Autodesk Inventor part; units mm, degrees
ref_plane "YZ Plane" through (0, 0, 0) normal (1, 0, 0) x (0, 1, 0)
ref_plane "XZ Plane" through (0, 0, 0) normal (0, 1, 0) x (-1, 0, 0)
ref_plane "XY Plane" through (0, 0, 0) normal (0, 0, 1) x (1, 0, 0)
sketch "Sketch1" plane through (0, 0, 0) normal (0, 0, 1) x (1, 0, 0)
  line L0 (0, 0) -> (127, 0)
  line L1 (127, 0) -> (127, 127)
  line L2 (127, 127) -> (0, 127)
  line L3 (0, 127) -> (0, 0)
  circle A0 centre (63.5, 63.5) radius 12.6844 construction
  circle A1 centre (9.4388, 90.7552) radius 3.175
  circle A2 centre (117.5612, 90.7552) radius 3.175
  circle A3 centre (117.5612, 36.2448) radius 3.175
  circle A4 centre (9.4388, 36.2448) radius 3.175
  line L4 (9.4388, 90.7552) -> (117.5612, 36.2448) construction
  line L5 (50.8, 50.8) -> (76.2, 50.8)
  line L6 (76.2, 50.8) -> (76.2, 76.2)
  line L7 (76.2, 76.2) -> (50.8, 76.2)
  line L8 (50.8, 76.2) -> (50.8, 50.8)
  line L9 (50.8, 50.8) -> (76.2, 76.2) construction
  line L10 (76.2, 50.8) -> (50.8, 76.2) construction
  point P0 (63.5, 127)
  point P1 (127, 63.5)
  dimension "d0" = 127
  dimension "d1" = 127
  dimension "d2" = 6.35
  dimension "d6" = 25.4
  dimension "d7" = 25.4
extrude "Extrusion1" add sketch "Sketch1" along normal blind 25.4
sketch "Sketch2" plane through (0, 0, 25.4) normal (0, 0, 1) x (1, 0, 0)
  line L0 (50.8, 50.8) -> (50.8, 76.2)
  line L1 (19.05, 76.2) -> (50.8, 76.2)
  line L2 (50.8, 76.2) -> (50.8, 69.85)
  line L3 (50.8, 69.85) -> (19.05, 69.85)
  line L4 (19.05, 69.85) -> (19.05, 76.2)
  line L5 (19.05, 57.15) -> (50.8, 57.15)
  line L6 (50.8, 57.15) -> (50.8, 50.8)
  line L7 (50.8, 50.8) -> (19.05, 50.8)
  line L8 (19.05, 50.8) -> (19.05, 57.15)
  line L9 (19.05, 67.31) -> (38.1, 67.31)
  line L10 (38.1, 67.31) -> (38.1, 59.69)
  line L11 (38.1, 59.69) -> (19.05, 59.69)
  line L12 (19.05, 59.69) -> (19.05, 67.31)
  line L13 (50.8, 76.2) -> (76.2, 76.2)
  line L14 (0, 127) -> (0, 0)
  line L15 (127, 127) -> (0, 127)
  line L16 (63.5, 127) -> (63.5, 0) construction
  line L17 (0, 0) -> (127, 0)
  line L18 (76.2, 50.8) -> (76.2, 76.2)
  line L19 (107.95, 76.2) -> (76.2, 76.2)
  line L20 (76.2, 76.2) -> (76.2, 69.85)
  line L21 (76.2, 69.85) -> (107.95, 69.85)
  line L22 (107.95, 69.85) -> (107.95, 76.2)
  line L23 (107.95, 57.15) -> (76.2, 57.15)
  line L24 (76.2, 57.15) -> (76.2, 50.8)
  line L25 (76.2, 50.8) -> (107.95, 50.8)
  line L26 (107.95, 50.8) -> (107.95, 57.15)
  line L27 (107.95, 67.31) -> (88.9, 67.31)
  line L28 (88.9, 67.31) -> (88.9, 59.69)
  line L29 (88.9, 59.69) -> (107.95, 59.69)
  line L30 (107.95, 59.69) -> (107.95, 67.31)
  line L31 (127, 127) -> (127, 0)
  point P0 (50.8, 76.2)
  dimension "d8" = 6.35
  dimension "d9" = 6.35
  dimension "d10" = 2.54
  dimension "d11" = 2.54
  dimension "d12" = 12.7
  dimension "d13" = 19.05
extrude "Extrusion2" cut sketch "Sketch2" against normal blind 25.4 contours L7 L8 L5 L0 | L23 L26 L25 L18 | L19 L22 L21 L18 | L3 L4 L1 L0 | L9 L10 L11 L12 | L30 L29 L28 L27
sketch "Sketch4" plane through (0, 0, 25.4) normal (0, 0, 1) x (1, 0, 0)
  line L0 (6.35, 82.55) -> (15.875, 82.55)
  line L1 (15.875, 82.55) -> (15.875, 44.45)
  line L2 (15.875, 44.45) -> (6.35, 44.45)
  line L3 (6.35, 44.45) -> (6.35, 82.55)
  line L4 (0, 127) -> (0, 0)
  line L5 (19.05, 69.85) -> (19.05, 76.2)
  line L6 (127, 127) -> (0, 127)
  line L7 (63.5, 127) -> (63.5, 0) construction
  line L8 (0, 0) -> (127, 0)
  line L9 (120.65, 82.55) -> (111.125, 82.55)
  line L10 (111.125, 82.55) -> (111.125, 44.45)
  line L11 (111.125, 44.45) -> (120.65, 44.45)
  line L12 (120.65, 44.45) -> (120.65, 82.55)
  line L13 (127, 127) -> (127, 0)
  line L14 (107.95, 69.85) -> (107.95, 76.2)
  point P0 (6.35, 63.5)
  point P1 (0, 63.5)
  point P2 (120.65, 63.5)
  dimension "d25" = 38.1
  dimension "d27" = 3.175
  dimension "d28" = 6.35
extrude "Extrusion4" cut sketch "Sketch4" against normal blind 25.4 contours L0 L1 L2 L3 | L12 L11 L10 L9
sketch "Sketch3" plane through (0, 0, 25.4) normal (0, 0, 1) x (1, 0, 0)
  line L0 (19.05, 50.8) -> (107.95, 50.8)
  line L1 (44.45, 50.8) -> (50.8, 50.8)
  line L2 (50.8, 50.8) -> (50.8, 19.05)
  line L3 (50.8, 19.05) -> (44.45, 19.05)
  line L4 (44.45, 19.05) -> (44.45, 50.8)
  line L5 (76.2, 50.8) -> (82.55, 50.8)
  line L6 (82.55, 50.8) -> (82.55, 19.05)
  line L7 (82.55, 19.05) -> (76.2, 19.05)
  line L8 (76.2, 19.05) -> (76.2, 50.8)
  line L9 (53.975, 38.1) -> (73.025, 38.1)
  line L10 (73.025, 38.1) -> (73.025, 19.05)
  line L11 (73.025, 19.05) -> (53.975, 19.05)
  line L12 (53.975, 19.05) -> (53.975, 38.1)
  line L13 (0, 0) -> (127, 0)
  line L14 (0, 127) -> (0, 0)
  line L15 (0, 63.5) -> (127, 63.5) construction
  line L16 (44.45, 76.2) -> (50.8, 76.2)
  line L17 (50.8, 76.2) -> (50.8, 107.95)
  line L18 (50.8, 107.95) -> (44.45, 107.95)
  line L19 (44.45, 107.95) -> (44.45, 76.2)
  line L20 (76.2, 76.2) -> (82.55, 76.2)
  line L21 (82.55, 76.2) -> (82.55, 107.95)
  line L22 (82.55, 107.95) -> (76.2, 107.95)
  line L23 (76.2, 107.95) -> (76.2, 76.2)
  line L24 (53.975, 88.9) -> (73.025, 88.9)
  line L25 (73.025, 88.9) -> (73.025, 107.95)
  line L26 (73.025, 107.95) -> (53.975, 107.95)
  line L27 (53.975, 107.95) -> (53.975, 88.9)
  point P0 (63.5, 19.05)
  point P1 (63.5, 50.8)
  point P2 (63.5, 107.95)
  point P3 (63.5, 76.2)
  dimension "d16" = 19.05
  dimension "d17" = 3.175
  dimension "d18" = 3.175
  dimension "d19" = 19.05
  dimension "d20" = 6.35
  dimension "d21" = 6.35
  dimension "d22" = 12.7
extrude "Extrusion3" cut sketch "Sketch3" against normal blind 25.4
sketch "Sketch5" plane through (0, 0, 25.4) normal (0, 0, 1) x (1, 0, 0)
  line L0 (41.275, 15.875) -> (85.725, 15.875)
  line L1 (85.725, 15.875) -> (85.725, 6.35)
  line L2 (85.725, 6.35) -> (41.275, 6.35)
  line L3 (41.275, 6.35) -> (41.275, 15.875)
  line L4 (0, 127) -> (0, 0)
  line L5 (0, 63.5) -> (127, 63.5) construction
  line L6 (127, 0) -> (127, 127)
  line L7 (73.025, 19.05) -> (53.975, 19.05)
  line L8 (0, 0) -> (127, 0)
  line L9 (41.275, 111.125) -> (85.725, 111.125)
  line L10 (85.725, 111.125) -> (85.725, 120.65)
  line L11 (85.725, 120.65) -> (41.275, 120.65)
  line L12 (41.275, 120.65) -> (41.275, 111.125)
  point P0 (63.5, 6.35)
  point P1 (63.5, 0)
  point P2 (63.5, 120.65)
  point P3 (63.5, 127)
  dimension "d31" = 3.175
  dimension "d32" = 6.35
  dimension "d33" = 44.45
extrude "Extrusion5" cut sketch "Sketch5" against normal blind 25.4
properties part number "BearingFlexure"
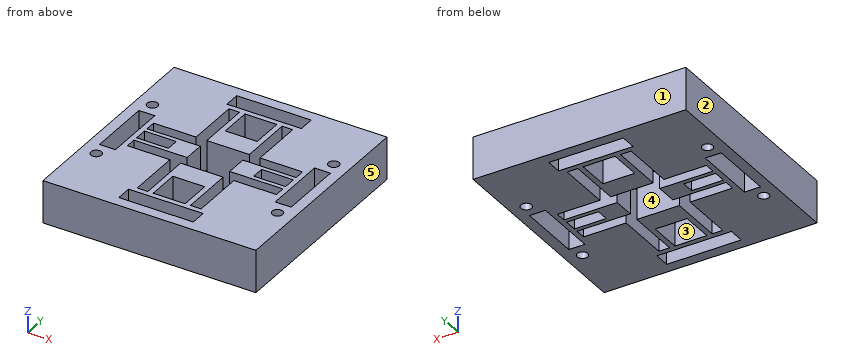
CAD build for the part. Positions are in the model's coordinates, mm. Face numbers are marked on the shaded views. A direction names the side the tool comes from. Round coordinates to 2 decimals unless told otherwise and drop trailing zeros. Write each loop counter-clockwise with the first axis right and the second up, starting at its lowest first coordinate (ties: lowest second). Pieces come first, ordered by that corner, then holes. Notation, with made-up numbers: (48.5, 36.5) -> (102.5, 36.5) arc R31 ccw to (102.5, 72.5) -> close; hole circle Ø4 at (34.5, 24). An arc over 180 degrees is marked (long way). Answer as a JSON object with one key per item and string values.
(1) Two-plate mould, pull along X, no slides. Class the marked faces 1, 2 and 3: +X half, -X half, draft (parallel to the pull), parting line (faces both ways), or undercut.
Reported:
{"face 1": "draft", "face 2": "-X half", "face 3": "undercut"}
(2) Probe probe 1 along X at (y, z) = (43, 21); probe 2 along Y at (x, z) = (62.5, 10) (3 decimals); probe 3 along Y at (x, z) = (29, 20). List the from-to ranges inside material, lowest first. Write a range as [from, to].
Reported:
{"probe 1": "x = [0, 44.45], [50.8, 76.2], [82.55, 127]", "probe 2": "y = [0, 6.35], [15.875, 19.05], [38.1, 50.8], [76.2, 88.9], [107.95, 111.125], [120.65, 127]", "probe 3": "y = [0, 50.8], [57.15, 59.69], [67.31, 69.85], [76.2, 127]"}
(3) Band-saw the part on D-D, the plane x = 21. List the corners of the cut face in (y, z).
Reported:
{"outline": "(0, 0) -> (50.8, 0) -> (50.8, 25.4) -> (0, 25.4) -> close; (57.15, 0) -> (59.69, 0) -> (59.69, 25.4) -> (57.15, 25.4) -> close; (67.31, 0) -> (69.85, 0) -> (69.85, 25.4) -> (67.31, 25.4) -> close; (76.2, 0) -> (127, 0) -> (127, 25.4) -> (76.2, 25.4) -> close"}
(4) Band-saw the part on A-A, the plane y = 63.5. List the corners of the cut face in (x, z) (3 decimals), then the cut area to 3 significant figures.
Reported:
{"outline": "(0, 0) -> (6.35, 0) -> (6.35, 25.4) -> (0, 25.4) -> close; (15.875, 0) -> (19.05, 0) -> (19.05, 25.4) -> (15.875, 25.4) -> close; (38.1, 0) -> (50.8, 0) -> (50.8, 25.4) -> (38.1, 25.4) -> close; (76.2, 0) -> (88.9, 0) -> (88.9, 25.4) -> (76.2, 25.4) -> close; (107.95, 0) -> (111.125, 0) -> (111.125, 25.4) -> (107.95, 25.4) -> close; (120.65, 0) -> (127, 0) -> (127, 25.4) -> (120.65, 25.4) -> close", "area": "1,130 mm^2"}
(5) Band-saw the part on C-C, the plane y = 99.5. List the corners of the cut face in (x, z) (3 decimals).
Reported:
{"outline": "(0, 0) -> (44.45, 0) -> (44.45, 25.4) -> (0, 25.4) -> close; (50.8, 0) -> (53.975, 0) -> (53.975, 25.4) -> (50.8, 25.4) -> close; (73.025, 0) -> (76.2, 0) -> (76.2, 25.4) -> (73.025, 25.4) -> close; (82.55, 0) -> (127, 0) -> (127, 25.4) -> (82.55, 25.4) -> close"}
(6) Which spindle directions (+Z, -Z, +X, -X, +Y, -Y) get a long thin tool onto all of the face, cutting with end or side? Do the marked faces 4 and 5. Say none if no direction does.
Reported:
{"face 4": "+Z, -Z", "face 5": "+Z, -Z, +X, +Y, -Y"}
